Geometry check sheet. Reference: the model listing, model coordinates, mm. A direction names the side the tool comes from. Round coordinates to 2 decimals unless told otherwise and drop trailing zeros. Loops run counter-clockwise (first coordinate to the right, second up) from the corner with the lowest first, then second, coordinate; pieces in that order, holes last. Notation, with made-up numbers: (46.5, 68.5) -> (84.5, 68.5) arc R19 cw to (84.5, 91.5) -> close; hole circle Ø3 at (13, -23.5). An arc over 180 degrees is marked (long way). Use a Markdown table: item, result. Add a question column.
Q1. Set-up check for faces 1 (the face through (-56.27, 1.23, -92.56)), 2 (the face through (-1.3, 2.5, -32.6)), 3 (the face through (-49.628, 1.232, 4.536)): record each of +Z, -Z, +X, -X, +Y, -Y from which the full face is reachable in a straight line by a thin tool's end or side.
Q2. Sectioned sample at C-C, the plane x = 32.5. Enter the section's corners in (y, z), then the cut area to 3 significant figures.
Q3. Sectioned sample at B-B, the plane y = 1.5. Give the number of separate pieces and of enclosed holes in the cut face, then the cut area to 3 significant figures.
Q4. Release check for a two-part mould opening along Z. For faces 4 (the face through (-1.3, 0, -32.6)), 5 (the face through (-63.22, 1.23, -95.2)), 6 (the face through (49.741, 1.232, 4.454)) record: released by +Z, released by -Z, zero draft, split by the parting line, or undercut.
Q5. Material ranges on L1, parallel to X at y = 0.85, z = -54; L2, parallel to X at y = 1.9, z = -72; L3, parallel to Z at x = -6, y = 0.95, recorded low to high.
Q6. Gauge pin test, flat ends, axial feed: P1, Ø1.2, axis at x = 11, y = 1.5, coming from the -Z side; P2, Ø0.8, axis at y = 1.5, z = -62.5, coming from the -X side; P3, Ø1.5, axis at y = 0.5, z = -16, coming from the -X side. Record the tip position at first contact, or that the pin passes through.
Q7. Sectioned sample at A-A, the plane x = 10. Enter the section's corners in (y, z).
```python
from build123d import *

# Parameters (mm, degrees)
SKETCH1_R           = 1.5
SKETCH1_W           = 5
SKETCH1_H           = 2.5
SKETCH1_W_2         = 2.5
SKETCH1_H_2         = 5
SKETCH1_W_3         = 24
SKETCH1_H_3         = 24
BOSS_EXTRUDE1_DEPTH = 2.5
FILLET1_R           = 3


with BuildPart() as part:
    # Sketch1 → Boss-Extrude1 (new body)
    with BuildSketch(Plane(origin=(0, 0, 0), x_dir=(1, 0, 0), z_dir=(0, 1, 0))):
        Polygon((42, 82.5), (42, 85), (35, 85), (35, 82.5), (28, 82.5), (28, 85), (21, 85), (21, 82.5), (14, 82.5), (14, 85), (7, 85), (7, 82.5), (-7, 82.5), (-7, 85), (-14, 85), (-14, 82.5), (-21, 82.5), (-21, 85), (-28, 85), (-28, 82.5), (-35, 82.5), (-35, 85), (-42, 85), (-42, 82.5), (-48.324658201, 82.5), (-55.266711269, 88.417765861), (-53.644883744, 90.320310336), (-58.972008275, 94.861427406), (-60.5938358, 92.958882931), (-65.92096033, 97.5), (-74.067282979, 97.5), (-74.067282979, 100), (-81.9, 100), (-81.9, 97.5), (-87.4, 97.5), (-87.4, 100), (-90, 100), (-90, 80), (-87.5, 80), (-87.5, 45), (-90, 45), (-90, 21.902362465), (-44.23398473, -11.580641316), (-25, -11.580641316), (-25, -9.080641316), (-15, -9.080641316), (-15, -11.580641316), (-5, -11.580641316), (-5, -9.080641316), (5, -9.080641316), (5, -11.580641316), (15, -11.580641316), (15, -9.080641316), (25, -9.080641316), (25, -11.580641316), (44.23398473, -11.580641316), (90, 21.902362465), (90, 45), (87.5, 45), (87.5, 80), (90, 80), (90, 100), (87.5, 100), (87.5, 97.5), (81.9, 97.5), (81.9, 100), (74.067282979, 100), (74.067282979, 97.5), (65.92096033, 97.5), (60.593835799, 92.958882931), (58.972008275, 94.861427406), (53.644883744, 90.320310336), (55.266711269, 88.417765861), (48.324658201, 82.5), align=None)
        Polygon((82.872162523, 22.882820213), (84.348313336, 20.865153546), (76.277646669, 14.960550296), (74.801495856, 16.978216962), align=None, mode=Mode.SUBTRACT)
        Polygon((67.558072522, 11.678835545), (69.034223335, 9.661168878), (60.963556668, 3.756565627), (59.487405855, 5.774232294), align=None, mode=Mode.SUBTRACT)
        Polygon((52.243982521, 0.474850877), (53.720133334, -1.54281579), (45.649466667, -7.447419041), (44.173315854, -5.429752374), align=None, mode=Mode.SUBTRACT)
        Polygon((-52.243982521, 0.474850877), (-44.173315854, -5.429752374), (-45.649466667, -7.447419041), (-53.720133334, -1.54281579), align=None, mode=Mode.SUBTRACT)
        Polygon((-59.487405855, 5.774232294), (-60.963556668, 3.756565627), (-69.034223335, 9.661168878), (-67.558072522, 11.678835545), align=None, mode=Mode.SUBTRACT)
        Polygon((-74.801495856, 16.978216962), (-76.277646669, 14.960550296), (-84.348313336, 20.865153546), (-82.872162523, 22.882820213), align=None, mode=Mode.SUBTRACT)
        with Locations(Location((-60, 18.419358684, 0), (0, 0, 270))):
            Circle(SKETCH1_R, mode=Mode.SUBTRACT)
        with Locations((-5, 27.75)):
            Rectangle(SKETCH1_W, SKETCH1_H, mode=Mode.SUBTRACT)
        with Locations((-15, 35)):
            Rectangle(SKETCH1_W_2, SKETCH1_H_2, mode=Mode.SUBTRACT)
        with Locations((5, 27.75)):
            Rectangle(SKETCH1_W, SKETCH1_H, mode=Mode.SUBTRACT)
        with Locations((15, 35)):
            Rectangle(SKETCH1_W_2, SKETCH1_H_2, mode=Mode.SUBTRACT)
        with Locations(Location((60, 18.419358684, 0), (0, 0, 270))):
            Circle(SKETCH1_R, mode=Mode.SUBTRACT)
        with Locations(Location((-60, 72, 0), (0, 0, 270))):
            Circle(SKETCH1_R, mode=Mode.SUBTRACT)
        with Locations((-15, 45)):
            Rectangle(SKETCH1_W_2, SKETCH1_H_2, mode=Mode.SUBTRACT)
        with Locations((-15, 55)):
            Rectangle(SKETCH1_W_2, SKETCH1_H_2, mode=Mode.SUBTRACT)
        with Locations((-5, 62.25)):
            Rectangle(SKETCH1_W, SKETCH1_H, mode=Mode.SUBTRACT)
        with Locations((0, 45)):
            Rectangle(SKETCH1_W_3, SKETCH1_H_3, mode=Mode.SUBTRACT)
        with Locations((15, 45)):
            Rectangle(SKETCH1_W_2, SKETCH1_H_2, mode=Mode.SUBTRACT)
        with Locations((15, 55)):
            Rectangle(SKETCH1_W_2, SKETCH1_H_2, mode=Mode.SUBTRACT)
        with Locations((5, 62.25)):
            Rectangle(SKETCH1_W, SKETCH1_H, mode=Mode.SUBTRACT)
        with Locations(Location((60, 72, 0), (0, 0, 270))):
            Circle(SKETCH1_R, mode=Mode.SUBTRACT)
    extrude(amount=BOSS_EXTRUDE1_DEPTH)

    # Fillet1
    fillet1_edges = [part.edges().sort_by_distance(p)[0] for p in [
        (90, 1.25, -21.902362465),
        (44.23398473, 1.25, 11.580641316),
        (-44.23398473, 1.25, 11.580641316),
        (-90, 1.25, -21.902362465),
    ]]
    fillet(fillet1_edges, radius=FILLET1_R)


solid = part.part
```
Values:
| question | item | result |
|---|---|---|
| 1 | face 1 | -Z, +Y, -Y |
| 1 | face 2 | +Z, -Z, +X, -X, +Y |
| 1 | face 3 | +Y, -Y |
| 2 | outline | (0, -82.5) -> (2.5, -82.5) -> (2.5, 11.58) -> (0, 11.58) -> close |
| 2 | area | 235 mm^2 |
| 3 | separate pieces | 1 |
| 3 | enclosed holes | 21 |
| 3 | area | 15,500 mm^2 |
| 4 | face 4 | zero draft |
| 4 | face 5 | released by -Z |
| 4 | face 6 | undercut |
| 5 | L1 | -87.5 to -16.25, -13.75 to -12, 12 to 13.75, 16.25 to 87.5 |
| 5 | L2 | -87.5 to -61.5, -58.5 to 58.5, 61.5 to 87.5 |
| 5 | L3 | -82.5 to -63.5, -61 to -57, -33 to -29, -26.5 to 11.58 |
| 6 | P1 | z = -85 |
| 6 | P2 | x = -87.5 |
| 6 | P3 | x = -82.96 |
| 7 | outline | (0, -85) -> (2.5, -85) -> (2.5, -57) -> (0, -57) -> close; (0, -33) -> (2.5, -33) -> (2.5, 11.58) -> (0, 11.58) -> close |
